Answer from the drawing. Dimensions are ordinates in mm from the lowest x, y and z of the part. A direction names the side the tool comes from. Give positions to 0.01 mm unless a question says otherwise; leave off trailing zeros. Loops run counter-clockwise (first coordinate to the right, second up) from the corner with the lowest first, then second, coordinate; pieces in that order, holes last. Notation, with made-up numbers: M 8.5,57.5 L 56.5,57.5 A23 cw 56.5,80.5 Z; hole C -32.5,-30.5 d10. An arc over 180 degrees is marked long. Use a Markdown table: item, result.
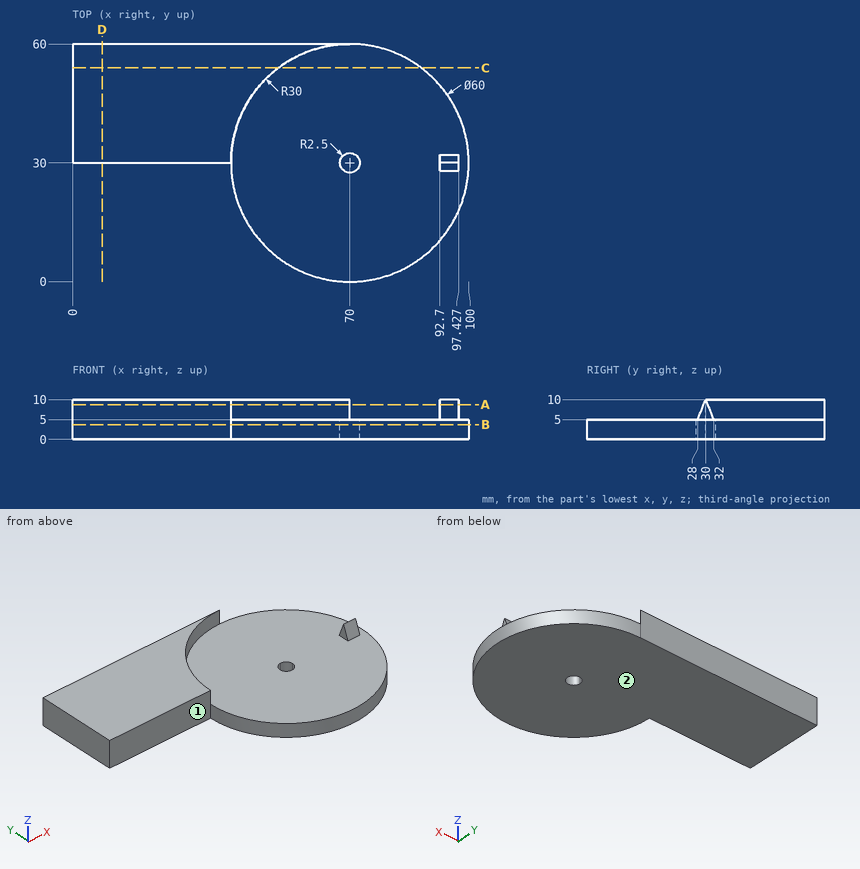
(1) A cutting plane is placed at D-D (x = 7.5). Write down the section's boundary in (y, z).
Entries:
| item | result |
|---|---|
| outline | M 30,0 L 60,0 L 60,10 L 30,10 Z |
(2) Given P1, Ø1.5, axis at y = 18, z = 5.5, coming from the +X side; P2, Ø3, axis at x = 29.5, z = 3.5, coming from the -Y side; P3, Ø4, axis at x = 79, z = 6, coming from the +Y side, each flat-ended and moving along its own axis, determine where each tip first touches the part or whether it passes through.
Entries:
| item | result |
|---|---|
| P1 | stops at x = 97.73 |
| P2 | stops at y = 30 |
| P3 | stops at y = 59.11 |
(3) A cutting plane is placed at A-A (z = 8.75). Write down the section's boundary in (x, y), and give its area (3 significant figures).
Entries:
| item | result |
|---|---|
| outline | M 0,30 L 40,30 A30 cw 70,60 L 0,60 Z; M 92.7,29.5 L 97.43,29.5 L 97.43,30.5 L 92.7,30.5 Z |
| area | 1,400 mm² |
(4) Which of the six approach directions +Z, -Z, +X, -X, +Y, -Y give full straight-line access (tool end or side, diameter ignored) to the marked faces 1 and 2?
Entries:
| item | result |
|---|---|
| face 1 | +Z, -Z, -X, -Y |
| face 2 | -Z, +X, -X, +Y, -Y |
(5) A cutting plane is placed at B-B (z = 3.75). Write down the section's boundary in (x, y), and give its area (3 significant figures).
Entries:
| item | result |
|---|---|
| outline | M 0,30 L 40,30 A30 ccw long 70,60 L 0,60 Z; hole C 70,30 d5 |
| area | 4,200 mm² |
(6) A cutting plane is placed at C-C (y = 54). Write down the section's boundary in (x, z).
Entries:
| item | result |
|---|---|
| outline | M 0,0 L 88,0 L 88,5 L 52,5 L 52,10 L 0,10 Z |
(7) Consider probe 1 along Y at (x, z) = (70, 4); probe 2 along Y at (x, z) = (21.5, 5); probe 3 along Z at (x, y) = (84, 27.5). Determine where each line is inside the solid, lowest interval first. Write a range as [from, to].
Entries:
| item | result |
|---|---|
| probe 1 | y = [0, 27.5], [32.5, 60] |
| probe 2 | y = [30, 60] |
| probe 3 | z = [0, 5] |
